from build123d import *

# Parameters (mm, degrees)
SKETCH1_W           = 130
SKETCH1_H           = 80
BOSS_EXTRUDE1_DEPTH = 2.8
SKETCH2_W           = 14.444444444
SKETCH2_H           = 2.8
SKETCH2_W_2         = 2.8
SKETCH2_H_2         = 13.333333334
SKETCH2_H_3         = 13.333333333
CUT_EXTRUDE1_DEPTH  = 153.669053839
CUT_EXTRUDE2_REACH  = 154.669
SKETCH3_R           = 1.7
CUT_EXTRUDE3_REACH  = 154.669


with BuildPart() as part:
    # Sketch1 → Boss-Extrude1 (new body)
    with BuildSketch(Plane.XY):
        with Locations((65, 40)):
            Rectangle(SKETCH1_W, SKETCH1_H)
    extrude(amount=BOSS_EXTRUDE1_DEPTH)

    # Sketch2 → Cut-Extrude1 (cut, through all)
    with BuildSketch(Plane.XY.offset(2.8)):
        with Locations((7.222222222, 1.4)):
            Rectangle(SKETCH2_W, SKETCH2_H)
        with Locations((36.111111111, 1.4)):
            Rectangle(SKETCH2_W, SKETCH2_H)
        with Locations((65, 1.4)):
            Rectangle(SKETCH2_W, SKETCH2_H)
        with Locations((93.888888889, 1.4)):
            Rectangle(SKETCH2_W, SKETCH2_H)
        Polygon((115.555555556, 0), (115.555555556, 2.8), (127.2, 2.8), (127.2, 13.333333333), (130, 13.333333333), (130, 0), align=None)
        with Locations((1.4, 20)):
            Rectangle(SKETCH2_W_2, SKETCH2_H_2)
        with Locations((1.4, 46.666666667)):
            Rectangle(SKETCH2_W_2, SKETCH2_H_3)
        with Locations((1.4, 73.333333334)):
            Rectangle(SKETCH2_W_2, SKETCH2_H_3)
        with Locations((128.6, 33.333333334)):
            Rectangle(SKETCH2_W_2, SKETCH2_H_3)
        with Locations((128.6, 60)):
            Rectangle(SKETCH2_W_2, SKETCH2_H_2)
    extrude(amount=-CUT_EXTRUDE1_DEPTH, mode=Mode.SUBTRACT)

    # Sketch3 → Cut-Extrude2 (cut, up to next)
    with BuildSketch(Plane.XY.offset(2.8), mode=Mode.PRIVATE) as cut_extrude2_sk1:
        with Locations((14.8, 74.5)):
            Circle(SKETCH3_R)
    cut_extrude2_tool1 = extrude(cut_extrude2_sk1.sketch, amount=-CUT_EXTRUDE2_REACH, mode=Mode.PRIVATE) & part.part
    # Sketch3 → Cut-Extrude2 (cut, up to next)
    with BuildSketch(Plane.XY.offset(2.8), mode=Mode.PRIVATE) as cut_extrude2_sk2:
        with Locations(Location((115.2, 74.5, 0), (0, 0, 180))):
            Circle(SKETCH3_R)
    cut_extrude2_tool2 = extrude(cut_extrude2_sk2.sketch, amount=-CUT_EXTRUDE2_REACH, mode=Mode.PRIVATE) & part.part
    add(cut_extrude2_tool1.solids().sort_by_distance((14.8, 74.5, 2.8))[0], mode=Mode.SUBTRACT)
    add(cut_extrude2_tool2.solids().sort_by_distance((115.2, 74.5, 2.8))[0], mode=Mode.SUBTRACT)

    # Sketch4 → Cut-Extrude3 (cut, up to next)
    with BuildSketch(Plane(origin=(0, 0, 0), x_dir=(-1, 0, 0), z_dir=(0, 0, -1)), mode=Mode.PRIVATE) as cut_extrude3_sk1:
        with BuildLine():
            Line((-29.625, 55.2), (-20.225, 55.2))
            ThreePointArc((-20.225, 55.2), (-19.158058262, 55.641941738), (-19.6, 54.575))
            Line((-19.6, 54.575), (-19.6, 23.425))
            ThreePointArc((-19.6, 23.425), (-19.158058262, 22.358058262), (-20.225, 22.8))
            Line((-20.225, 22.8), (-29.625, 22.8))
            ThreePointArc((-29.625, 22.8), (-30.691941738, 22.358058262), (-30.25, 23.425))
            Line((-30.25, 23.425), (-30.25, 54.575))
            ThreePointArc((-30.25, 54.575), (-30.691941738, 55.641941738), (-29.625, 55.2))
        make_face()
    cut_extrude3_tool1 = extrude(cut_extrude3_sk1.sketch, amount=-CUT_EXTRUDE3_REACH, mode=Mode.PRIVATE) & part.part
    add(cut_extrude3_tool1.solids().sort_by_distance((24.925, 39, 0))[0], mode=Mode.SUBTRACT)


solid = part.part
Build history of the part. All positions in model axes, mm. A direction names the side the tool comes from. Coordinates: 2 decimals unless noted, no trailing zeros. Order: outer loops, then holes, each group sorted by start corner. A loop starts at its lowest first (then second) coordinate and runs counter-clockwise, first axis right, second up. Notation, with made-up numbers: M 70.25,10 L 102.25,10 A18 ccw 102.25,32 Z; hole C 48.5,-11 d5. An arc over 180 degrees is marked long. One line per question, with ' | ' between items. Start each with the question number.
Q1. Saw through at A-A (y = 36). List the corners of the cut face in (x, z).
Q2. Saw through at C-C (y = 12). List the corners of the cut face in (x, z), then the cut area to 3 significant figures.
Q3. Saw through at B-B (y = 74.5). List the corners of the cut face in (x, z).
Q4. Flat gauge pins, fed straight in: pin 1 Ø1 at (x, y) = (19.6, 22.8) entering from +Z; pin 2 Ø1.4 at (y, z) = (31, 2) entering from +X; pin 3 Ø3 at (x, y) = (53.5, 45.5) entering from -Z; pin 4 Ø0.8 at (x, z) = (5, 1) entering from -Y. Where does each tip first touch, or does it go through?
Q5. Saw through at D-D (z = 2.1). Count the separate pieces of the cut face and the enclosed holes in it, then the cut area to 3 significant figures.
Q6. Two-plate mould, pull along X, no slides. Class faces 1 (the face through (25, 55.2, 1)), 2 (the face through (115.556, 1, 1)), 3 (the face through (101.111, 1, 1)), 4 (the face through (79, 0, 1)): +X half, -X half, draft (parallel to the pull), parting line (faces both ways), or undercut.
Q7. Probe L1, parallel to X at y = 74.5, z = 1.2; L2, parallel to X at y = 22.5, z = 0.5; L3, parallel to X at y = 52, z = 1.3. List the from-to ranges inside material, lowest first. Write a range as from..to.
Q8. 3-axis set-ups, long thin cutter, end or side, ignore diameter. For faces 5 (the face through (1, 40, 1)), 6 (the face through (129, 53.333, 1)), 7 (the face through (28.889, 1, 1)): which of +Z, -Z, +X, -X, +Y, -Y reach the whole face in a straight line?
Check values:
1) outline: M 0,0 L 19.6,0 L 19.6,2.8 L 0,2.8 Z; M 30.25,0 L 127.2,0 L 127.2,2.8 L 30.25,2.8 Z
2) outline: M 0,0 L 127.2,0 L 127.2,2.8 L 0,2.8 Z | area: 356 mm2
3) outline: M 2.8,0 L 13.1,0 L 13.1,2.8 L 2.8,2.8 Z; M 16.5,0 L 113.5,0 L 113.5,2.8 L 16.5,2.8 Z; M 116.9,0 L 130,0 L 130,2.8 L 116.9,2.8 Z
4) pin 1: passes through | pin 2: stops at x = 127.2 | pin 3: stops at z = 0 | pin 4: stops at y = 2.8
5) separate pieces: 1 | enclosed holes: 3 | area: 9,610 mm2
6) face 1: undercut | face 2: +X half | face 3: undercut | face 4: draft
7) L1: x = 2.8..13.1, 16.5..113.5, 116.9..130 | L2: x = 2.8..19.05, 20.15..29.7, 30.8..130 | L3: x = 2.8..19.6, 30.25..130
8) face 5: +Z, -Z, -X | face 6: +Z, -Z, +X | face 7: +Z, -Z, -Y
